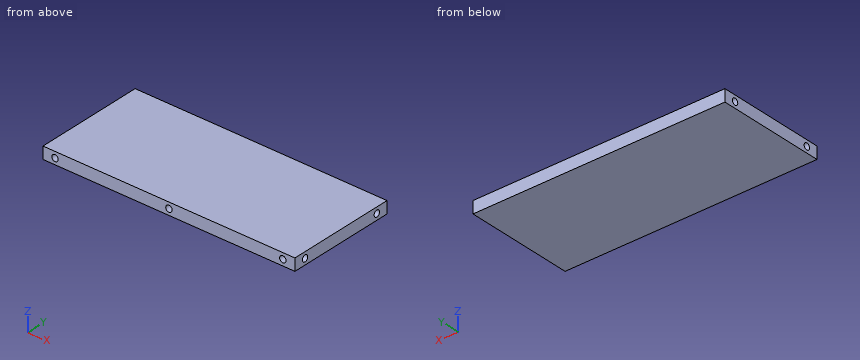
from build123d import *

# Parameters (mm, degrees)
SKETCH1_W               = 314
SKETCH1_H               = 136
BOSS_EXTRUDE1_DEPTH     = 15
SKETCH2_R               = 4
CUT_EXTRUDE1_DEPTH      = 10
LPATTERN2_COUNT         = 2
LPATTERN2_PITCH         = 106
MIRROR1_COPY_1_SKETCH_R = 4
MIRROR1_COPY_1_DEPTH    = 10
SKETCH3_R               = 4
CUT_EXTRUDE2_DEPTH      = 10
LPATTERN1_COUNT         = 3
LPATTERN1_PITCH         = 142


with BuildPart() as part:
    # Sketch1 → Boss-Extrude1 (new body)
    with BuildSketch(Plane.XY):
        Rectangle(SKETCH1_W, SKETCH1_H)
    extrude(amount=BOSS_EXTRUDE1_DEPTH)

    # Sketch2 → Cut-Extrude1 (cut)
    with BuildSketch(Plane.ZY.offset(157)):
        with Locations((7.5, 53)):
            Circle(SKETCH2_R)
    cut_extrude1 = extrude(amount=-CUT_EXTRUDE1_DEPTH, mode=Mode.SUBTRACT)

    # LPattern2: Cut-Extrude1 ×2
    with Locations(*[(0, -i * LPATTERN2_PITCH, 0) for i in range(1, LPATTERN2_COUNT)]):
        add(cut_extrude1, mode=Mode.SUBTRACT)

    # Mirror1: Cut-Extrude1 across plane
    add(cut_extrude1.mirror(Plane(origin=(0, 0, 0), x_dir=(0, 0, 1), z_dir=(1, 0, 0))), mode=Mode.SUBTRACT)

    # Mirror1 copy 1 sketch → Mirror1 copy 1 (cut)
    with BuildSketch(Plane(origin=(157, -106, 0), x_dir=(0, 0, 1), z_dir=(1, 0, 0))):
        with Locations((7.5, -53)):
            Circle(MIRROR1_COPY_1_SKETCH_R)
    extrude(amount=-MIRROR1_COPY_1_DEPTH, mode=Mode.SUBTRACT)

    # Sketch3 → Cut-Extrude2 (cut)
    with BuildSketch(Plane.XZ.offset(68)):
        with Locations((-142, 7.5)):
            Circle(SKETCH3_R)
    cut_extrude2 = extrude(amount=-CUT_EXTRUDE2_DEPTH, mode=Mode.SUBTRACT)

    # LPattern1: Cut-Extrude2 ×3
    with Locations(*[(i * LPATTERN1_PITCH, 0, 0) for i in range(1, LPATTERN1_COUNT)]):
        add(cut_extrude2, mode=Mode.SUBTRACT)


solid = part.part
Part model, mm, in its own coordinate system. Coordinates: 2 decimals unless noted, no trailing zeros. Loops run counter-clockwise (first coordinate to the right, second up) from the corner with the lowest first, then second, coordinate; pieces in that order, holes last. Notation, with made-up numbers: M -29.75,28.25 L 2.25,28.25 A25 cw 2.25,52.25 Z; hole C 83,44.25 d9. An arc over 180 degrees is marked long. Use a Markdown table: item, result. Add a question column.
Q1. Cut at A-A (x = 0). Write the cut outline in (y, z), and give its area (3 significant figures).
Q2. Pin check, flat tips, straight feed: P1, Ø6.5, axis at x = 0, z = 7.5, coming from the -Y side; P2, Ø5, axis at y = -53, z = 7.5, coming from the +X side; P3, Ø4, axis at y = -54.5, z = 8.5, coming from the -X side. Stop position of each tip, or through.
Q3. Cut at B-B (y = -53). Write the cut outline in (x, z).
Q4. Probe L1, parallel to Y at x = 154.5, z = 7.5; L2, parallel to Z at x = 142, y = -64.5. List the from-to ranges inside material, lowest first.
Worked out:
| question | item | result |
|---|---|---|
| 1 | outline | M -68,0 L 68,0 L 68,15 L -68,15 L -68,11.5 L -58,11.5 L -58,3.5 L -68,3.5 Z |
| 1 | area | 1,960 mm2 |
| 2 | P1 | stops at y = -58 |
| 2 | P2 | stops at x = 147 |
| 2 | P3 | stops at x = -147 |
| 3 | outline | M -157,0 L 157,0 L 157,3.5 L 147,3.5 L 147,11.5 L 157,11.5 L 157,15 L -157,15 L -157,11.5 L -147,11.5 L -147,3.5 L -157,3.5 Z |
| 4 | L1 | y = -68 to -57, -49 to 49, 57 to 68 |
| 4 | L2 | z = 0 to 3.5, 11.5 to 15 |
